Here's how the part is built. I have some questions about the finished solid (model axes, mm). Give positions to 0.01 mm unless a question says otherwise; leave off trailing zeros. Loops run counter-clockwise (first coordinate to the right, second up) from the corner with the lowest first, then second, coordinate; pieces in that order, holes last. Notation, with made-up numbers: M 81.25,11 L 86.25,11 A15 cw 86.25,18 Z; hole C 51,-5 d6. An arc over 180 degrees is marked long. Answer as CSV lines item,"result". Start each with the question number.
Item 1: I want a section at C-C on y = 12. List the corners of the cut face in (x, z) for me.
Item 2: I want a section at A-A on z = 3. Give the number of separate pieces and of enclosed holes in the cut face, plus the area to 3 significant figures.
Item 3: Will these pins go through, and if not, where does the flat tip stop? P1, Ø6.5, axis at x = -95, y = 0, coming from the +Z side; P2, Ø3, axis at x = -75, y = 0, coming from the +Z side.
Item 4: If I drill on line 1 along Y through (x, z) = (-75, 4); line 2 along X through (y, z) = (2, 6.25); line 3 along X through (y, z) = (1.5, 0.5), over which ranges is the centre line in solid material (lowest first)? Write a range as from..to.
Item 5: I want a section at B-B on x = -75. List the corners of the cut face in (y, z) for me, plus the area to 3 significant figures.
from build123d import *

# Parameters (mm, degrees)
BOSS_EXTRUDE1_DEPTH   = 6.4
F_5_0MM_DOWEL_HOLE1_D = 5
FILLET1_R             = 19.05
CUT_EXTRUDE1_REACH    = 128.605
SKETCH9_R             = 5


with BuildPart() as part:
    # Sketch1 → Boss-Extrude1 (new body)
    with BuildSketch(Plane.XY):
        Polygon((-120, 19.05), (125, 19.05), (125, -19.05), (-120, -19.05), (-125, -14.05), (-125, 14.05), align=None)
    extrude(amount=BOSS_EXTRUDE1_DEPTH)

    # Ø5.0mm Dowel Hole1 (through all)
    with Locations(Plane.XY.offset(6.4)):
        with Locations((-75, 0), (-95, 0)):
            Hole(F_5_0MM_DOWEL_HOLE1_D / 2)

    # Fillet1
    fillet1_edges = [part.edges().sort_by_distance(p)[0] for p in [
        (125, -19.05, 3.2),
        (125, 19.05, 3.2),
    ]]
    fillet(fillet1_edges, radius=FILLET1_R - 0.0001)  # a hair under: the kernel refuses the full size

    # Sketch9 → Cut-Extrude1 (cut, up to next)
    with BuildSketch(Plane.XY.offset(6.4), mode=Mode.PRIVATE) as cut_extrude1_sk1:
        with Locations((105.95, 0)):
            Circle(SKETCH9_R)
    cut_extrude1_tool1 = extrude(cut_extrude1_sk1.sketch, amount=-CUT_EXTRUDE1_REACH, mode=Mode.PRIVATE) & part.part
    add(cut_extrude1_tool1.solids().sort_by_distance((105.95, 0, 6.4))[0], mode=Mode.SUBTRACT)


solid = part.part
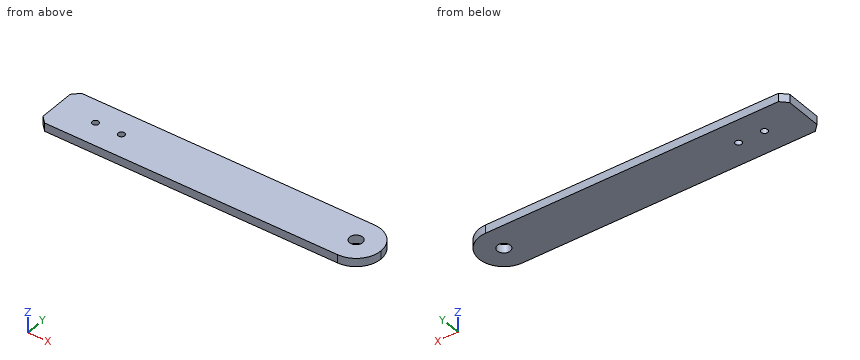
Result:
1,outline,"M -125,0 L 120.75,0 L 120.75,6.4 L -125,6.4 Z"
2,separate pieces,"1"
2,enclosed holes,"3"
2,area,"9,230 mm^2"
3,P1,"z = 6.4"
3,P2,"through"
4,line 1,"-19.05..-2.5, 2.5..19.05"
4,line 2,"-125..-96.5, -93.5..-76.5, -73.5..101.37, 110.53..124.89"
4,line 3,"-125..-97, -93..-77, -73..101.18, 110.72..124.94"
5,outline,"M -19.05,0 L -2.5,0 L -2.5,6.4 L -19.05,6.4 Z; M 2.5,0 L 19.05,0 L 19.05,6.4 L 2.5,6.4 Z"
5,area,"212 mm^2"
